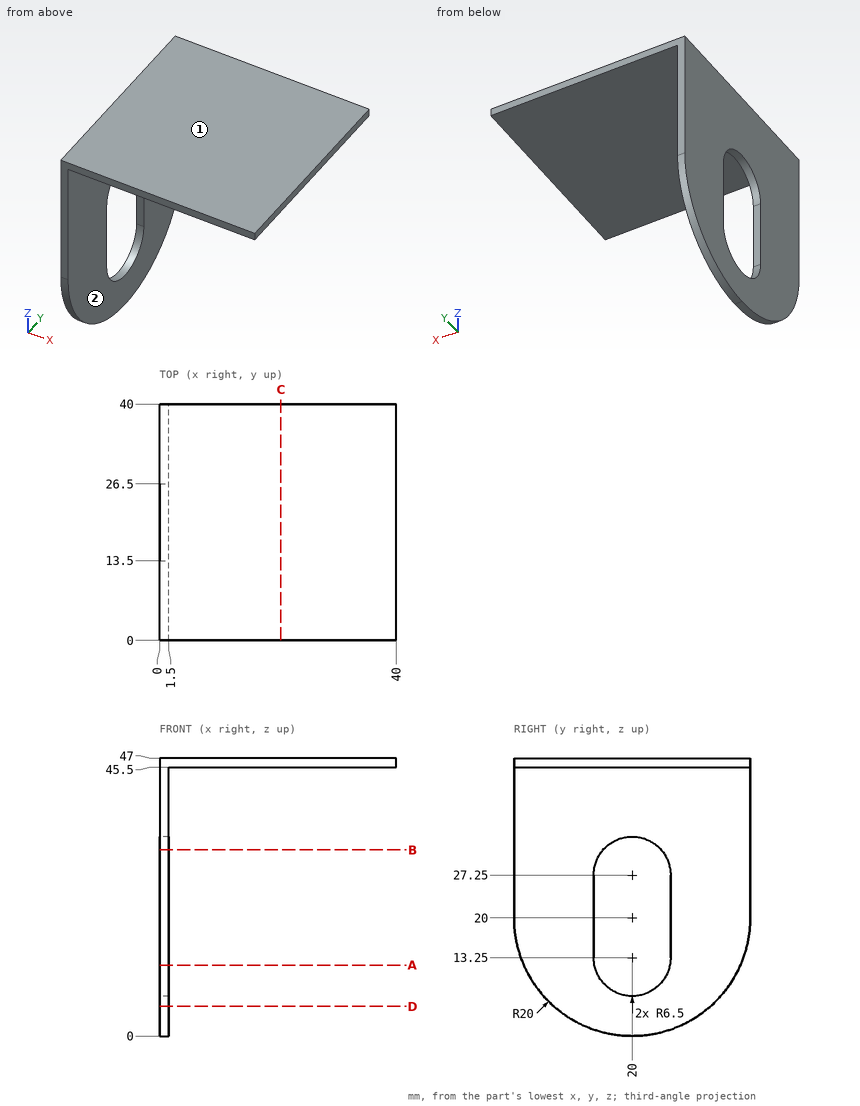
Check sheet for the drawn part. Datum: minimum x, y, z corner. Units: mm. A direction names the side the tool comes from. Round coordinates to 2 decimals unless told otherwise and drop trailing zeros. Order: outer loops, then holes, each group sorted by start corner. A loop starts at its lowest first (then second) coordinate and runs counter-clockwise, first axis right, second up.
(1) Cross-section at C-C, the plane x = 20.5. Enter the section's corners in (y, z).
(2) Cross-section at B-B, the plane z = 31.5. Enter the section's corners in (x, y).
(3) Scan lines: probe 1 along Z at (x, y) = (37, 11.5); probe 2 along X at (y, z) = (32, 37). Record each from-to range of solid material in increasing order.
(4) Cross-section at D-D, the plane z = 5. Enter the section's corners in (x, y), and give its area (3 significant figures).
(5) Go/stop test with flat-tipped pins: P1, Ø1, axis at y = 7, z = 14.5, coming from the +X side; P2, Ø5, axis at x = 23, y = 34, coming from the -Z side; P3, Ø1.6, axis at x = 1, z = 17.5, coming from the +Y side; P4, Ø6, axis at y = 28, z = 5.5, coming from the -X side. Record where each tip stops, or that it passes through.
(6) Cross-section at A-A, the plane z = 12. Enter the section's corners in (x, y), and give its area (3 significant figures).
(7) Access from +Z, -Z, +X, -X, +Y, -Y to the whole of each face (thin tool, end or side, straight path). Record for the marked faces 1 and 2.
Check sheet entries:
1. outline: (0, 45.5) - (40, 45.5) - (40, 47) - (0, 47) - close
2. outline: (0, 0) - (1.5, 0) - (1.5, 15.08) - (0, 15.08) - close; (0, 24.92) - (1.5, 24.92) - (1.5, 40) - (0, 40) - close
3. probe 1: z = 45.5 to 47
3. probe 2: x = 0 to 1.5
4. outline: (0, 6.77) - (1.5, 6.77) - (1.5, 33.23) - (0, 33.23) - close
4. area: 39.7 mm2
5. P1: stops at x = 1.5
5. P2: stops at z = 45.5
5. P3: stops at y = 39.93
5. P4: stops at x = 0
6. outline: (0, 1.67) - (1.5, 1.67) - (1.5, 13.62) - (0, 13.62) - close; (0, 26.38) - (1.5, 26.38) - (1.5, 38.33) - (0, 38.33) - close
6. area: 35.9 mm2
7. face 1: +Z, +X, -X, +Y, -Y
7. face 2: -Z, +X, +Y, -Y
